Could you check a few things on this model? Use its own coordinates, in mm. Give positions to 0.01 mm unless a question says otherwise; leave off trailing zeros. Loops run counter-clockwise (first coordinate to the right, second up) from the corner with the lowest first, then second, coordinate; pieces in that order, holes last. Notation, with made-up numbers: (-8, 58) - (25, 58) arc R10 ccw to (25, 70) - close; hole circle Ø10 at (83, 44.5). An arc over 180 degrees is marked (long way). Write each question's results on one line, items separated by ' | '. Start each with the question number.
1) I want a section at A-A, the plane y = 171.5. Write out the boundary of the cut face in (x, z).
2) If we mould it in two halves opening along Z, with no side actions, what happens to faces 1 (the face through (-3, 4, 5)), 2 (the face through (234.964, 235.742, 2.535)), 3 (the face through (-3, 4, 0))? For each: +Z half, -Z half, draft (parallel to the pull), parting line (faces both ways), or undercut.
3) I'm going to push flat-ended pins straight in: pin 1 (4 mm diameter, centred on x = -126.875, y = -179.4, fed in from +Z); pin 2 (6 mm diameter, centred on x = -126.875, y = -150.6, fed in from -Z). Where does each tip first touch, or does it pass through?
4) I want a section at B-B, the plane z = 4.2. Count the separate pieces of the cut face and the enclosed holes in it, and give its area (3 significant figures).
5) If I drill on probe 1 along X at (y, z) = (-179.4, 1.1) (3 decimals); probe 2 along X at (y, z) = (104.5, 3.25); probe 3 along Y at (x, z) = (145, 1.95), over which ranges is the centre line in solid material (lowest first)? Write a range as [from, to].
from build123d import *

# Parameters (mm, degrees)
SKETCH1_W           = 500
SKETCH1_H           = 500
SKETCH1_R           = 2.5
SKETCH1_W_2         = 50
SKETCH1_H_2         = 140
BOSS_EXTRUDE1_DEPTH = 5
CUT_EXTRUDE1_START  = -5
SKETCH2_R           = 2.5
CUT_EXTRUDE1_DEPTH  = 5
FILLET1_R           = 10
FILLET2_R           = 50
SKETCH3_W           = 10
SKETCH3_H           = 20
CUT_EXTRUDE2_DEPTH  = 354.588744165


with BuildPart() as part:
    # Sketch1 → Boss-Extrude1 (new body)
    with BuildSketch(Plane.XY):
        Rectangle(SKETCH1_W, SKETCH1_H)
        with Locations((127, 147.5)):
            Circle(SKETCH1_R, mode=Mode.SUBTRACT)
        with Locations((127, 132.5)):
            Circle(SKETCH1_R, mode=Mode.SUBTRACT)
        with Locations((145, 132.5)):
            Circle(SKETCH1_R, mode=Mode.SUBTRACT)
        with Locations((145, 147.5)):
            Circle(SKETCH1_R, mode=Mode.SUBTRACT)
        with Locations((-145, 147.5)):
            Circle(SKETCH1_R, mode=Mode.SUBTRACT)
        with Locations((-145, 132.5)):
            Circle(SKETCH1_R, mode=Mode.SUBTRACT)
        with Locations((-127, 132.5)):
            Circle(SKETCH1_R, mode=Mode.SUBTRACT)
        with Locations((-127, 147.5)):
            Circle(SKETCH1_R, mode=Mode.SUBTRACT)
        with Locations((183, 140)):
            Rectangle(SKETCH1_W_2, SKETCH1_H_2, mode=Mode.SUBTRACT)
        with Locations((-183, 140)):
            Rectangle(SKETCH1_W_2, SKETCH1_H_2, mode=Mode.SUBTRACT)
    extrude(amount=BOSS_EXTRUDE1_DEPTH)

    # Sketch2 → Cut-Extrude1 (cut)
    with BuildSketch(Plane.XY.offset(5).offset(CUT_EXTRUDE1_START)):
        with Locations((-145, 132.5)):
            Circle(SKETCH2_R)
        with Locations((-163.125, -150.6)):
            Circle(SKETCH2_R)
        with Locations((-126.875, -150.6)):
            Circle(SKETCH2_R)
        with Locations((-126.875, -179.4)):
            Circle(SKETCH2_R)
        with Locations((-163.125, -179.4)):
            Circle(SKETCH2_R)
        with Locations((-145, -115)):
            Circle(SKETCH2_R)
        with Locations((-145, -215)):
            Circle(SKETCH2_R)
        with Locations((145, -215)):
            Circle(SKETCH2_R)
        with Locations((145, -115)):
            Circle(SKETCH2_R)
        with Locations((163.125, -179.4)):
            Circle(SKETCH2_R)
        with Locations((126.875, -179.4)):
            Circle(SKETCH2_R)
        with Locations((126.875, -150.6)):
            Circle(SKETCH2_R)
        with Locations((163.125, -150.6)):
            Circle(SKETCH2_R)
    extrude(amount=CUT_EXTRUDE1_DEPTH, mode=Mode.SUBTRACT)

    # Fillet1
    fillet1_edges = [part.edges().sort_by_distance(p)[0] for p in [
        (-208, 70, 2.5),
        (-158, 70, 2.5),
        (-158, 210, 2.5),
        (-208, 210, 2.5),
        (158, 70, 2.5),
        (208, 70, 2.5),
        (208, 210, 2.5),
        (158, 210, 2.5),
    ]]
    fillet(fillet1_edges, radius=FILLET1_R)

    # Fillet2
    fillet2_edges = [part.edges().sort_by_distance(p)[0] for p in [
        (250, -250, 2.5),
        (-250, -250, 2.5),
        (-250, 250, 2.5),
        (250, 250, 2.5),
    ]]
    fillet(fillet2_edges, radius=FILLET2_R)

    # Sketch3 → Cut-Extrude2 (cut, through all)
    with BuildSketch(Plane.XY.offset(5)):
        with Locations((-92, 140)):
            Rectangle(SKETCH3_W, SKETCH3_H)
        with BuildLine():
            ThreePointArc((-97, 150), (-92, 155), (-87, 150))
            Line((-87, 150), (-97, 150))
        make_face()
        with BuildLine():
            Line((-97, 130), (-87, 130))
            ThreePointArc((-87, 130), (-92, 125), (-97, 130))
        make_face()
        with BuildLine():
            ThreePointArc((97, 130), (92, 125), (87, 130))
            Line((87, 130), (87, 150))
            ThreePointArc((87, 150), (92, 155), (97, 150))
            Line((97, 150), (97, 130))
        make_face()
    extrude(amount=-CUT_EXTRUDE2_DEPTH, mode=Mode.SUBTRACT)


solid = part.part
Answers:
1) outline: (-250, 0) - (-208, 0) - (-208, 5) - (-250, 5) - close; (-158, 0) - (158, 0) - (158, 5) - (-158, 5) - close; (208, 0) - (250, 0) - (250, 5) - (208, 5) - close
2) face 1: +Z half | face 2: draft | face 3: -Z half
3) pin 1: passes through | pin 2: stops at z = 0
4) separate pieces: 1 | enclosed holes: 24 | area: 233,000 mm2
5) probe 1: x = [-250, -165.625], [-160.625, -129.375], [-124.375, 124.375], [129.375, 160.625], [165.625, 250] | probe 2: x = [-250, -208], [-158, 158], [208, 250] | probe 3: y = [-250, -217.5], [-212.5, -117.5], [-112.5, 130], [135, 145], [150, 250]
